For this review, take the finished solid that the model builds, in its own axes (mm). A direction names the side the tool comes from. Round coordinates to 2 decimals unless told otherwise and drop trailing zeros. Loops run counter-clockwise (first coordinate to the right, second up) from the corner with the lowest first, then second, coordinate; pieces in that order, holes last. Notation, with made-up numbers: M -14.5,26.25 L -7.5,26.25 A31 ccw -7.5,57.25 Z; hole C 41.5,-33 d2. An arc over 180 degrees is marked long. One line per question, with ' | ' between items. Start each with the question number.
1) We need section A-A (x = -10.5). Give the boundary of the cut face in (y, z), and give its area (3 significant figures).
2) We need section D-D (z = 6.5). Give the boundary of the cut face in (x, y), and give its area (3 significant figures).
3) For pin 1 Ø2 at (x, y) = (6.5, 3) entering from -Z; pin 2 Ø10 at (x, z) = (2.5, 13) entering from -Y; pin 3 Ø6 at (x, z) = (7.5, 11) entering from +Y, all flat-tipped, find the tip position at first contact; note any pin that passes through.
4) For probe 1 along Z at (x, y) = (-6.5, 2.25); probe 2 along X at (y, z) = (-0.75, 6); probe 3 along X at (y, z) = (1.5, 5.25), list the stretches that pass through material, from the lowest coordinate up. Write a range as from..to.
5) We need section C-C (x = -7). Give the boundary of the cut face in (y, z), and give its area (3 significant figures).
6) Mouldability with a two-part tool opening along X and no side actions: class faces 1 (the face through (-9, 0, 8)), 2 (the face through (-8.998, 0.088, 16.746)), 3 (the face through (-7, 0, -0.5)) as pulls with the +X half, pulls with the -X half, needs draft (parallel to the pull), parting line crosses it, or undercut.
7) For faces 4 (the face through (5, 0, 8)), 5 (the face through (-0.049, -3.695, 15.514)), 6 (the face through (-8.998, 0.088, -0.254)), 7 (the face through (-13.097, 0.191, 0.986)), 8 (the face through (5.002, 0.088, 16.746)), list the 3-axis set-ups (+Z, -Z, +X, -X, +Y, -Y) from which the entire face can be reached by the end or side of a thin tool; tool diameter is ignored.
```python
from build123d import *

# Parameters (mm, degrees)
CROQUIS1_R                   = 2
SALIENTE_EXTRUIR1_DEPTH      = 2
SALIENTE_EXTRUIR2_DEPTH      = 15
SALIENTE_EXTRUIR2_DEPTH_BACK = 2.5
CROQUIS2_R                   = 2


with BuildPart() as part:
    # Croquis1 → Saliente-Extruir1 (new body)
    with BuildSketch(Plane.XY):
        with BuildLine():
            ThreePointArc((-3.250445743, 4.811532279), (-13.1, 0), (-3.250445743, -4.811532279))
            ThreePointArc((-3.250445743, -4.811532279), (0, -3.694574334), (3.250445743, -4.811532279))
            ThreePointArc((3.250445743, -4.811532279), (13.1, 0), (3.250445743, 4.811532279))
            ThreePointArc((3.250445743, 4.811532279), (0, 3.694574334), (-3.250445743, 4.811532279))
        make_face()
        with Locations((-7, 0)):
            Circle(CROQUIS1_R, mode=Mode.SUBTRACT)
        with Locations(Location((7, 0, 0), (0, 0, 180))):
            Circle(CROQUIS1_R, mode=Mode.SUBTRACT)
    saliente_extruir1 = extrude(amount=SALIENTE_EXTRUIR1_DEPTH)

    # Croquis2 → Saliente-Extruir2 (add, two sides: drawn at the far end of the back side and taken through both)
    with BuildSketch(Plane.XY.offset(2).offset(-SALIENTE_EXTRUIR2_DEPTH_BACK)):
        with Locations((7, 0)):
            Circle(CROQUIS2_R)
        with Locations((-7, 0)):
            Circle(CROQUIS2_R)
    extrude(amount=SALIENTE_EXTRUIR2_DEPTH + SALIENTE_EXTRUIR2_DEPTH_BACK)

    # Simetría1: Saliente-Extruir1 across plane
    add(saliente_extruir1.mirror(Plane.XY.offset(8.25)))


solid = part.part
```
Answers below:
1) outline: M -5,0 L 5,0 L 5,2 L -5,2 Z; M -5,14.5 L 5,14.5 L 5,16.5 L -5,16.5 Z | area: 40.0 mm^2
2) outline: C -7,0 d4; C 7,0 d4 | area: 25.1 mm^2
3) pin 1: z = 0 | pin 2: y = -6.1 | pin 3: y = 2
4) probe 1: 0..2, 14.5..16.5 | probe 2: -8.85..-5.15, 5.15..8.85 | probe 3: -8.32..-5.68, 5.68..8.32
5) outline: M -6.1,0 L -2,0 L -2,-0.5 L 2,-0.5 L 2,0 L 6.1,0 L 6.1,2 L 2,2 L 2,14.5 L 6.1,14.5 L 6.1,16.5 L 2,16.5 L 2,17 L -2,17 L -2,16.5 L -6.1,16.5 L -6.1,14.5 L -2,14.5 L -2,2 L -6.1,2 Z | area: 103 mm^2
6) face 1: undercut | face 2: undercut | face 3: needs draft
7) face 4: none | face 5: +Z, -Z, -Y | face 6: -Z | face 7: +Z, -Z | face 8: +Z
